```python
from build123d import *

# Parameters (mm, degrees)
SKETCH_1_R             = 3
EXTRUDE_1_DEPTH        = 41
HOLE_WIZARD_M3_1_D     = 2.5
HOLE_WIZARD_M3_1_DEPTH = 8.5
HOLE_WIZARD_M3_1_TIP   = 0.751075774
HOLE_WIZARD_M3_2_D     = 2.5
HOLE_WIZARD_M3_2_DEPTH = 8.5
HOLE_WIZARD_M3_2_TIP   = 0.751075774


with BuildPart() as part:
    # 草图1 → 凸台-拉伸1 (new body)
    with BuildSketch(Plane(origin=(0, 0, 0), x_dir=(1, 0, 0), z_dir=(0, 1, 0))):
        Circle(SKETCH_1_R)
    extrude(amount=EXTRUDE_1_DEPTH)

    # M3 螺纹孔1
    with Locations(Plane.ZX.offset(41)):
        with Locations((0, 0)):
            Hole(HOLE_WIZARD_M3_1_D / 2, depth=HOLE_WIZARD_M3_1_DEPTH)
            with Locations((0, 0, -(HOLE_WIZARD_M3_1_DEPTH + HOLE_WIZARD_M3_1_TIP / 2))):  # 118° drill point
                Cone(0, HOLE_WIZARD_M3_1_D / 2, HOLE_WIZARD_M3_1_TIP, mode=Mode.SUBTRACT)

    # M3 螺纹孔2
    with Locations(Plane(origin=(0, 0, 0), x_dir=(0, 0, -1), z_dir=(0, -1, 0))):
        with Locations((0, 0)):
            Hole(HOLE_WIZARD_M3_2_D / 2, depth=HOLE_WIZARD_M3_2_DEPTH)
            with Locations((0, 0, -(HOLE_WIZARD_M3_2_DEPTH + HOLE_WIZARD_M3_2_TIP / 2))):  # 118° drill point
                Cone(0, HOLE_WIZARD_M3_2_D / 2, HOLE_WIZARD_M3_2_TIP, mode=Mode.SUBTRACT)


solid = part.part
```
Geometry: final body of the model. Coordinates: model frame, mm. A direction names the side the tool comes from. Coordinates: 2 decimals unless noted, no trailing zeros. Order: outer loops, then holes, each group sorted by start corner. A loop starts at its lowest first (then second) coordinate and runs counter-clockwise, first axis right, second up. Notation, with made-up numbers: (45.25, 28.25) - (61.25, 28.25) arc R8 ccw to (61.25, 41.25) - close; hole circle Ø8 at (64, -38). An arc over 180 degrees is marked (long way). Write each question's results on one line, items separated by ' | '.
1) Section C-C, the plane x = 2.6. Return loops of the section in (y, z), plus the area to 3 significant figures.
Results list:
outline: (0, -1.5) - (41, -1.5) - (41, 1.5) - (0, 1.5) - close | area: 123 mm^2
2) Section D-D, the plane z = -2.3. Return loops of the section in (x, y), plus the area to 3 significant figures.
Results list:
outline: (-1.93, 0) - (1.93, 0) - (1.93, 41) - (-1.93, 41) - close | area: 158 mm^2
3) Pull-direction query (Z, two-part tool) for faces 1 (the cylindrical face through (-3, 20, 0)), 2 (the flat face through (1, 41, 1)), 3 (the conical face through (-0.21, 9.12, 0.05)); classes: pulls with the +Z half, pulls with the -Z half, needs draft (parallel to the pull), parting line crosses it, or undercut.
Results list:
face 1: parting line crosses it | face 2: needs draft | face 3: undercut
4) Section B-B, the plane y = 25. Return loops of the section in (x, z).
Results list:
outline: circle Ø6 at (0, 0)
5) Pin query (flat end, axial travel): pin 1 (2 mm diameter, centred on x = 2, y = 13.5, fed in from +Z). Return the tip coordinate at first contact, or that it passes through.
Results list:
pin 1: z = 2.83
6) Section A-A, the plane y = 35.5. Return loops of the section in (x, z), plus the area to 3 significant figures.
Results list:
outline: circle Ø6 at (0, 0); hole circle Ø2.5 at (0, 0) | area: 23.4 mm^2
7) Line query: line 1 (X direction, y = 34.5, z = 0); line 2 (Z direction, x = -0.95, y = 2). Output: solid intervals per line, ascending. Write a range as from..to.
Results list:
line 1: -3..-1.25, 1.25..3 | line 2: -2.85..-0.81, 0.81..2.85
8) Set-up query: faces 4 (the flat face through (1, 0, 1)), 5 (the cylindrical face through (-1.22, 36.69, 0.27)), 6 (the cylindrical face through (-1.22, 4.31, -0.27)). Return all of +Z, -Z, +X, -X, +Y, -Y with unobstructed straight access to the full face (end or side cutting, diameter ignored); none if empty.
Results list:
face 4: +Z, -Z, +X, -X, -Y | face 5: +Y | face 6: -Y
